Read the model definition and answer for the solid it produces. Units are mm, in the model's axes. A direction names the side the tool comes from. Coordinates: 2 decimals unless noted, no trailing zeros. Loops run counter-clockwise (first coordinate to the right, second up) from the corner with the lowest first, then second, coordinate; pieces in that order, holes last. Notation, with made-up numbers: M -13,62 L 4,62 A14 cw 4,81 Z; hole C 10.5,-0.75 d2. An arc over 180 degrees is marked long. Put each result on its own line as item: value.
from build123d import *

# Parameters (mm, degrees)
SKETCH1_W             = 42.7
SKETCH1_H             = 42.7
BOSS_EXTRUDE1_DEPTH   = 34
SKETCH2_R             = 11
BOSS_EXTRUDE2_DEPTH   = 2
SKETCH3_R             = 3.175
CUT_EXTRUDE1_DEPTH    = 47.985582895
M3_TAPPED_HOLE1_D     = 2.5
M3_TAPPED_HOLE1_DEPTH = 7.5
M3_TAPPED_HOLE1_TIP   = 0.751075774
CHAMFER1_SIZE         = 5


with BuildPart() as part:
    # Sketch1 → Boss-Extrude1 (new body)
    with BuildSketch(Plane(origin=(0, 0, 0), x_dir=(1, 0, 0), z_dir=(0, 1, 0))):
        Rectangle(SKETCH1_W, SKETCH1_H)
    extrude(amount=BOSS_EXTRUDE1_DEPTH)

    # Sketch2 → Boss-Extrude2 (add)
    with BuildSketch(Plane(origin=(0, 34, 0), x_dir=(1, 0, 0), z_dir=(0, 1, 0))):
        with Locations(Location((0, 0, 0), (0, 0, 270))):
            Circle(SKETCH2_R)
    extrude(amount=BOSS_EXTRUDE2_DEPTH)

    # Sketch3 → Cut-Extrude1 (cut, through all)
    with BuildSketch(Plane(origin=(0, 36, 0), x_dir=(1, 0, 0), z_dir=(0, 1, 0))):
        with Locations(Location((0, 0, 0), (0, 0, 270))):
            Circle(SKETCH3_R)
    extrude(amount=-CUT_EXTRUDE1_DEPTH, mode=Mode.SUBTRACT)

    # M3 Tapped Hole1
    with Locations(Plane(origin=(0, 34, 0), x_dir=(1, 0, 0), z_dir=(0, 1, 0))):
        with Locations((15.5, 15.5), (-15.5, -15.5), (-15.5, 15.5), (15.5, -15.5)):
            Hole(M3_TAPPED_HOLE1_D / 2, depth=M3_TAPPED_HOLE1_DEPTH)
            with Locations((0, 0, -(M3_TAPPED_HOLE1_DEPTH + M3_TAPPED_HOLE1_TIP / 2))):  # 118° drill point
                Cone(0, M3_TAPPED_HOLE1_D / 2, M3_TAPPED_HOLE1_TIP, mode=Mode.SUBTRACT)

    # Chamfer1
    chamfer1_edges = [part.edges().sort_by_distance(p)[0] for p in [
        (21.35, 17, 21.35),
        (-21.35, 17, 21.35),
        (-21.35, 17, -21.35),
        (21.35, 17, -21.35),
    ]]
    chamfer(chamfer1_edges, length=CHAMFER1_SIZE)


solid = part.part
1) Find section C-C, the plane z = -5.5. Write down the section's boundary in (x, y).
Answer list:
outline: M -21.35,0 L 21.35,0 L 21.35,34 L 9.53,34 L 9.53,36 L -9.53,36 L -9.53,34 L -21.35,34 Z
2) Given pin 1 Ø4 at (x, z) = (-15.5, 15.5) entering from +Y; pin 2 Ø8 at (x, z) = (-10.5, -10) entering from -Y; pin 3 Ø5.5 at (x, z) = (0, 0) entering from +Y, each flat-ended and moving along its own axis, determine where each tip first touches the part or whether it passes through.
Answer list:
pin 1: stops at y = 34
pin 2: stops at y = 0
pin 3: passes through
3) Which of the six approach directions +Z, -Z, +X, -X, +Y, -Y give full straight-line access (tool end or side, diameter ignored) to faces 1 (the flat face through (-5, 34, -10)), 2 (the flat face through (0, 17, 21.35))?
Answer list:
face 1: +Y
face 2: +Z, +X, -X, +Y, -Y
4) Find section D-D, the plane x = 12. Write down the section's boundary in (y, z).
Answer list:
outline: M 0,-21.35 L 34,-21.35 L 34,21.35 L 0,21.35 Z
5) Find section B-B, the plane y = 15.5. Write down the section's boundary in (x, z) (3 decimals), plus the area to 3 significant figures.
Answer list:
outline: M -21.35,-16.35 L -16.35,-21.35 L 16.35,-21.35 L 21.35,-16.35 L 21.35,16.35 L 16.35,21.35 L -16.35,21.35 L -21.35,16.35 Z; hole C 0,0 d6.35
area: 1,740 mm^2
6) Find section A-A, the plane z = 0. Write down the section's boundary in (x, y) (3 decimals), plus the area to 3 significant figures.
Answer list:
outline: M -21.35,0 L -3.175,0 L -3.175,36 L -11,36 L -11,34 L -21.35,34 Z; M 3.175,0 L 21.35,0 L 21.35,34 L 11,34 L 11,36 L 3.175,36 Z
area: 1,270 mm^2
7) Straight lines are drawn through the part: line 1 (X direction, y = 31.75, z = -15.5); line 2 (Z direction, x = -15, y = 31). For each, find the intervals that lie inside material, in ascending order. Write a range as [from, to].
Answer list:
line 1: x = [-21.35, -16.75], [-14.25, 14.25], [16.75, 21.35]
line 2: z = [-21.35, -16.65], [-14.35, 14.35], [16.65, 21.35]
8) Determine the mould class of faces 3 (the flat face through (-21.35, 17, 0)), 4 (the flat face through (21.35, 17, 0)), 5 (the cylindrical face through (15.66, 30.2, 14.26)), 6 (the cylindrical face through (-15.34, 30.2, 14.26)) for opening direction X: released by +X, released by -X, zero draft, split by the parting line, or undercut.
Answer list:
face 3: released by -X
face 4: released by +X
face 5: undercut
face 6: undercut
